from build123d import *

# Parameters (mm, degrees)
SKETCH1_R           = 17.5
BOSS_EXTRUDE1_DEPTH = 415
CUT_EXTRUDE1_REACH  = 832.369
SKETCH2_R           = 6.5
SKETCH3_W           = 10
SKETCH3_H           = 317.5
BOSS_EXTRUDE2_DEPTH = 20
FILLET1_R           = 20
SKETCH4_R           = 6.5
CUT_EXTRUDE2_DEPTH  = 542


with BuildPart() as part:
    # Sketch1 → Boss-Extrude1 (new, symmetric)
    with BuildSketch(Plane.XY):
        Circle(SKETCH1_R)
    extrude(amount=BOSS_EXTRUDE1_DEPTH, both=True)

    # Sketch2 → Cut-Extrude1 (cut, up to next)
    with BuildSketch(Plane.XY.offset(415), mode=Mode.PRIVATE) as cut_extrude1_sk1:
        Circle(SKETCH2_R)
    cut_extrude1_tool1 = extrude(cut_extrude1_sk1.sketch, amount=-CUT_EXTRUDE1_REACH, mode=Mode.PRIVATE) & part.part
    add(cut_extrude1_tool1.solids().sort_by_distance((0, 0, 415))[0], mode=Mode.SUBTRACT)

    # Sketch3 → Boss-Extrude2 (add, symmetric)
    with BuildSketch(Plane(origin=(0, 0, 0), x_dir=(0, 0, -1), z_dir=(1, 0, 0))):
        with Locations((-215, -158.75)):
            Rectangle(SKETCH3_W, SKETCH3_H)
        with Locations((215, -158.75)):
            Rectangle(SKETCH3_W, SKETCH3_H)
    extrude(amount=BOSS_EXTRUDE2_DEPTH, both=True)

    # Fillet1
    fillet1_edges = [part.edges().sort_by_distance(p)[0] for p in [
        (-20, -317.5, -215),
        (20, -317.5, -215),
        (-20, -317.5, 215),
        (20, -317.5, 215),
    ]]
    fillet(fillet1_edges, radius=FILLET1_R - 0.0001)  # a hair under: the kernel refuses the full size

    # Sketch4 → Cut-Extrude2 (cut)
    with BuildSketch(Plane.XY.offset(220)):
        with Locations(Location((0, -292.5, 0), (0, 0, 270))):
            Circle(SKETCH4_R)
    extrude(amount=-CUT_EXTRUDE2_DEPTH, mode=Mode.SUBTRACT)


solid = part.part
Read the model definition and answer for the solid it produces. Units are mm, in the model's axes. A direction names the side the tool comes from. Round coordinates to 2 decimals unless told otherwise and drop trailing zeros. Write each loop counter-clockwise with the first axis right and the second up, starting at its lowest first coordinate (ties: lowest second). Pieces come first, ordered by that corner, then holes. Notation, with made-up numbers: (75, 87) - (112, 87) arc R20 cw to (112, 121) - close; hole circle Ø2 at (-18, 7). An arc over 180 degrees is marked (long way). One line per question, with ' | ' between items. Start each with the question number.
1. Section A-A (y = -176) is taken. Determine the outline of the cut face in (x, z).
2. Section B-B (z = 310.5) is taken. Determine the outline of the cut face in (x, y).
3. For faces 1 (the face through (-13.986, -311.797, -215.07)), 2 (the face through (-13.887, -10.648, 5.81)), determine the directions among +Z, -Z, +X, -X, +Y, -Y from which every point of the face is accessible in a straight line to the end or side of a thin tool.
4. For a pull along Z with two mould halves and no side action, classify faces 3 (the face through (14.297, -311.486, 214.93)), 4 (the face through (0, -161, -210)), 5 (the face through (0, -8, -415)), 6 (the face through (0, -161, 210)) as +Z half, -Z half, draft (parallel to the pull), parting line (faces both ways), or undercut.
5. Find the intervals of material crossed by probe 1 along Y at (x, z) = (-0.5, -57); probe 2 along Z at (x, y) = (-6, -124); probe 3 along X at (y, z) = (-292, -213), in increasing order. Write a range as [from, to].
6. Each of these flat-tipped pins is pushed along its axis until it touches: pin 1 (2 mm diameter, centred on x = 0.5, y = -3, fed in from +Z); pin 2 (2 mm diameter, centred on x = 14.5, z = 85, fed in from -Y); pin 3 (7 mm diameter, centred on x = -2, y = -2, fed in from -Z); pin 4 (8 mm diameter, centred on x = 0, y = -292.5, fed in from +Z). Where does it stop, or does it pass through?
Filled in:
1) outline: (-20, -220) - (20, -220) - (20, -210) - (-20, -210) - close; (-20, 210) - (20, 210) - (20, 220) - (-20, 220) - close
2) outline: circle Ø35 at (0, 0); hole circle Ø13 at (0, 0)
3) face 1: +Z, -Z, -X, -Y | face 2: none
4) face 3: draft | face 4: undercut | face 5: -Z half | face 6: undercut
5) probe 1: [-17.49, -6.48], [6.48, 17.49] | probe 2: [-220, -210], [210, 220] | probe 3: [-20, -6.48], [6.48, 20]
6) pin 1: z = 220 | pin 2: y = -11.14 | pin 3: z = -220 | pin 4: through
